Can you work these out from the model? Positions are in its coordinate system, mm. A direction names the side the tool comes from. Give positions to 0.01 mm unless a question says otherwise; leave off trailing zeros. Loops run counter-clockwise (first coordinate to the right, second up) from the corner with the lowest first, then second, coordinate; pieces in that order, holes last. Notation, with made-up numbers: M -29.75,13.25 L -13.75,13.25 A22 cw -13.75,25.25 Z; hole C 43,25.25 d7. An arc over 180 degrees is marked long. Put each result on its own line as item: value. Start each with the question number.
1) If we mould it in two halves opening along X, with no side actions, what happens to faces 4 (the cylindrical face through (-23.43, -2.47, 7.4)), 5 (the flat face through (-19, -0.5, 2)), 6 (the cylindrical face through (-20.326, -2.472, 4.692)), 7 (the cylindrical face through (23.4, -2.53, 0.57))? For each: +X half, -X half, draft (parallel to the pull), parting line (faces both ways), or undercut.
2) Imagine slicing it at B-B (x = 0). Write out the boundary of the cut face in (y, z).
3) Imagine slicing it at C-C (y = 0). Write out the boundary of the cut face in (x, z), then the cut area to 3 significant figures.
4) For faces 1 (the flat face through (-17, -4.5, 4)), 2 (the flat face through (17.5, -4.5, 4.8)), 3 (the flat face through (0, -7.922, 4)), which set-ups out of +Z, -Z, +X, -X, +Y, -Y let a thin tool reach every point of the face, with its end or its side?
5) Please list where these lines run through material, in increasing order: line 1 along X through (y, z) = (-1.75, 4); line 2 along X through (y, z) = (-3.55, 4); line 3 along Y through (x, z) = (19.5, 2). Write a range as from..to.
6) For P1, Ø3, axis at x = -3, y = -8, coming from the -Z side; P2, Ø1, axis at y = 9.5, z = 1.5, coming from the -X side; P3, Ø1, axis at x = 15, z = 4, coming from the +Y side; P4, Ø3, axis at y = -7.5, z = 1, coming from the -X side, each with a flat end and sliding along its axis, tell me the tip position at first contact or that it passes through.
7) Imagine slicing it at D-D (z = 6.75). Write out the boundary of the cut face in (x, y) (3 decimals).
8) Imagine slicing it at A-A (z = 4). Write out the boundary of the cut face in (x, y) (3 decimals).
from build123d import *

# Parameters (mm, degrees)
SALIENTE_EXTRUIR1_DEPTH = 8
CORTAR_EXTRUIR1_DEPTH   = 29.91366459
CROQUIS3_R              = 1.5
CORTAR_EXTRUIR2_DEPTH   = 5
REDONDEO1_R             = 2


with BuildPart() as part:
    # Croquis1 → Saliente-Extruir1 (new body)
    with BuildSketch(Plane.XY):
        with BuildLine():
            Line((-24, -0.5), (-13.99106858, -0.5))
            ThreePointArc((-13.99106858, -0.5), (0, 14), (13.99106858, -0.5))
            Line((13.99106858, -0.5), (24, -0.5))
            Line((24, -0.5), (24, -4.5))
            Line((24, -4.5), (13.257073584, -4.5))
            ThreePointArc((13.257073584, -4.5), (0, -14), (-13.257073584, -4.5))
            Line((-13.257073584, -4.5), (-24, -4.5))
            Line((-24, -4.5), (-24, -0.5))
        make_face()
    extrude(amount=SALIENTE_EXTRUIR1_DEPTH)

    # Croquis2 → Cortar-Extruir1 (cut, through all)
    with BuildSketch(Plane.XY.offset(8)):
        with BuildLine():
            Line((-6.425, 7.922081482), (6.425, 7.922081482))
            ThreePointArc((6.425, 7.922081482), (10.2, 0), (6.425, -7.922081482))
            Line((6.425, -7.922081482), (-6.425, -7.922081482))
            ThreePointArc((-6.425, -7.922081482), (-10.2, 0), (-6.425, 7.922081482))
        make_face()
    extrude(amount=-CORTAR_EXTRUIR1_DEPTH, mode=Mode.SUBTRACT)

    # Croquis3 → Cortar-Extruir2 (cut)
    with BuildSketch(Plane(origin=(0, -0.5, 0), x_dir=(1, 0, 0), z_dir=(0, 1, 0))):
        with Locations(Location((18.99553429, -4, 0), (0, 0, 270))):
            Circle(CROQUIS3_R)
        with Locations(Location((-18.99553429, -4, 0), (0, 0, 270))):
            Circle(CROQUIS3_R)
    extrude(amount=-CORTAR_EXTRUIR2_DEPTH, mode=Mode.SUBTRACT)

    # Redondeo1
    redondeo1_edges = [part.edges().sort_by_distance(p)[0] for p in [
        (-24, -2.5, 8),
        (24, -2.5, 8),
        (24, -2.5, 0),
        (-24, -2.5, 0),
    ]]
    fillet(redondeo1_edges, radius=REDONDEO1_R)


solid = part.part
Recorded:
1. face 4: -X half
1. face 5: draft
1. face 6: undercut
1. face 7: +X half
2. outline: M -14,0 L -7.92,0 L -7.92,8 L -14,8 Z; M 7.92,0 L 14,0 L 14,8 L 7.92,8 Z
3. outline: M -14,0 L -10.2,0 L -10.2,8 L -14,8 Z; M 10.2,0 L 14,0 L 14,8 L 10.2,8 Z
3. area: 60.8 mm²
4. face 1: +Z, -Z, -X, -Y
4. face 2: +Z, -Z, +X, -Y
4. face 3: +Z, -Z
5. line 1: -24..-20.5, -17.5..-10.05, 10.05..17.5, 20.5..24
5. line 2: -24..-20.5, -17.5..-9.56, 9.56..17.5, 20.5..24
5. line 3: -4.5..-0.5
6. P1: z = 0
6. P2: x = -10.72
6. P3: y = -0.5
6. P4: x = -12.65
7. outline: M -23.854,-4.5 L -13.257,-4.5 A14 ccw 13.257,-4.5 L 23.854,-4.5 L 23.854,-0.5 L 13.991,-0.5 A14 ccw long -13.991,-0.5 L -23.854,-0.5 Z; hole M -6.425,-7.922 L 6.425,-7.922 A10.2 ccw 6.425,7.922 L -6.425,7.922 A10.2 ccw Z
8. outline: M -24,-4.5 L -20.496,-4.5 L -20.496,-0.5 L -24,-0.5 Z; M -17.496,-4.5 L -13.257,-4.5 A14 ccw 13.257,-4.5 L 17.496,-4.5 L 17.496,-0.5 L 13.991,-0.5 A14 ccw long -13.991,-0.5 L -17.496,-0.5 Z; M 20.496,-4.5 L 24,-4.5 L 24,-0.5 L 20.496,-0.5 Z; hole M -6.425,-7.922 L 6.425,-7.922 A10.2 ccw 6.425,7.922 L -6.425,7.922 A10.2 ccw Z
